Study the drawing (mm; zero at the part's minimum x, y, z) and answer. A direction names the side the tool comes from. Round coordinates to 2 decimals unless told otherwise and drop trailing zeros. Write each loop counter-clockwise with the first axis right and the second up, starting at its lowest first coordinate (ties: lowest second). Pieces come first, ordered by that corner, then holes.
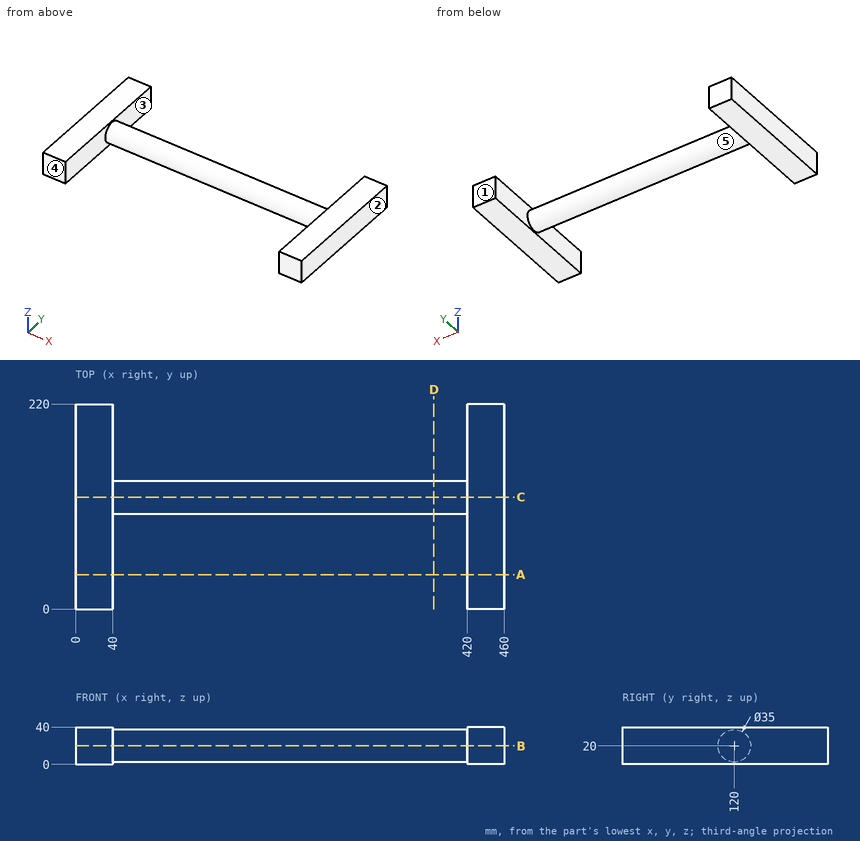
Q1. Find the intervals of material crossed by L1, parallel to X at y = 174.5, z = 12; L2, parallel to Z at x = 365, y = 121.5; L3, parallel to Z at x = 94, y = 113, in increasing order.
Q2. Find section B-B (z = 20). Determine the outline of the cut face in (x, y), plus the area to 3 significant figures.
Q3. A tool of negligible diameter and unlimited length cuts with its end or side. For the marked faces 4 and 5, from which of +Z, -Z, +X, -X, +Y, -Y can it reach the whole face along a straight path? Write none if from no direction.
Q4. The mould has two halves that part along X. Classify the marked faces 1, 2 and 3: +X half, -X half, draft (parallel to the pull), parting line (faces both ways), or undercut.
Q5. Find section D-D (x = 384.5). Determine the outline of the cut face in (y, z).
Q6. Given pin 1 (2 mm diameter, centred on x = 177, z = 12, fed in from -Y); pin 2 (1.5 mm diameter, centred on x = 406, z = 16, fed in from +Y), each flat-ended and moving along its own axis, determine where each tip first touches the part or whether it passes through.
Q7. Find section A-A (y = 37). Determine the outline of the cut face in (x, z).
Q8. Find section C-C (y = 120). Determine the outline of the cut face in (x, z).
Report:
1. L1: x = 0 to 40, 420 to 460
1. L2: z = 2.56 to 37.44
1. L3: z = 3.96 to 36.04
2. outline: (0, 0) - (40, 0) - (40, 102.5) - (420, 102.5) - (420, 0) - (460, 0) - (460, 220) - (420, 220) - (420, 137.5) - (40, 137.5) - (40, 220) - (0, 220) - close
2. area: 30,900 mm2
3. face 4: +Z, -Z, +X, -X, -Y
3. face 5: none
4. face 1: draft
4. face 2: +X half
4. face 3: undercut
5. outline: circle Ø35 at (120, 20)
6. pin 1: stops at y = 103.96
6. pin 2: stops at y = 137.2
7. outline: (0, 0) - (40, 0) - (40, 40) - (0, 40) - close; (420, 0) - (460, 0) - (460, 40) - (420, 40) - close
8. outline: (0, 0) - (40, 0) - (40, 2.5) - (420, 2.5) - (420, 0) - (460, 0) - (460, 40) - (420, 40) - (420, 37.5) - (40, 37.5) - (40, 40) - (0, 40) - close
